Check sheet for the modelled part. Datum: model origin and axes. Units: mm. A direction names the side the tool comes from. Give positions to 0.01 mm unless a question says otherwise; leave off trailing zeros. Order: outer loops, then holes, each group sorted by start corner. A loop starts at its lowest first (then second) coordinate and runs counter-clockwise, first axis right, second up. Notation, with made-up numbers: (-31, 85.25) -> (-18, 85.25) arc R13 cw to (-18, 97.25) -> close; hole circle Ø6 at (12, 36). An arc over 180 degrees is marked (long way). One line per question, with ' | ' between items.
```python
from build123d import *

# Parameters (mm, degrees)
F0_W     = 25
F0_H     = 25
F1_DEPTH = 8.3
F2_R     = 5
F3_DEPTH = 4
F5_DEPTH = 25


with BuildPart() as f1:
    # F0 (on Top) → F1 (new body)
    with BuildSketch(Plane.XY):
        Rectangle(F0_W, F0_H)
    extrude(amount=F1_DEPTH)

    # F2 (on face) → F3 (join)
    with BuildSketch(Plane.XY.offset(8.3)):
        Circle(F2_R)
    extrude(amount=F3_DEPTH)

    # F4 (on face) → F5 (cut)
    with BuildSketch(Plane.XY.offset(8.3)):
        Polygon((12.5, -12.5), (12.5, 0), (0, -12.5), align=None)
    extrude(amount=-F5_DEPTH, mode=Mode.SUBTRACT)


solid = f1.part
```
Q1. Section check B-B (x = -3.5). Enter the section's corners in (y, z).
Result sheet:
outline: (-12.5, 0) -> (12.5, 0) -> (12.5, 8.3) -> (3.57, 8.3) -> (3.57, 12.3) -> (-3.57, 12.3) -> (-3.57, 8.3) -> (-12.5, 8.3) -> close
Q2. Access from +Z, -Z, +X, -X, +Y, -Y to the whole of each face (thin tool, end or side, straight path). Record for faces 1 (the face through (0, 0, 0)), 2 (the face through (-1.08, -4.88, 10.27)).
Result sheet:
face 1: -Z, +X, -X, +Y, -Y | face 2: +Z
Q3. Thickness scan on line 1 (Z direction, x = -0.25, y = -10.25); line 2 (X direction, y = -3.25, z = 9.25); line 3 (Y direction, x = 3, z = 8.25). Record the ranges inside material, lowest first.
Result sheet:
line 1: z = 0 to 8.3 | line 2: x = -3.8 to 3.8 | line 3: y = -9.5 to 12.5
Q4. Section check A-A (z = 4.75). Enter the section's corners in (x, y), and give its area (3 significant figures).
Result sheet:
outline: (-12.5, -12.5) -> (0, -12.5) -> (12.5, 0) -> (12.5, 12.5) -> (-12.5, 12.5) -> close | area: 547 mm2
Q5. Section check C-C (y = 10.75). Enter the section's corners in (x, z), and give its area (4 significant figures).
Result sheet:
outline: (-12.5, 0) -> (12.5, 0) -> (12.5, 8.3) -> (-12.5, 8.3) -> close | area: 207.5 mm2
Q6. Depth check by flat-ended pin: pin 1 Ø1.5 at (y, z) = (-9.5, 6) entering from +X; pin 2 Ø1 at (x, z) = (1.5, 10.5) entering from +Y. Enter the tip coordinate at first touch or a pass-through.
Result sheet:
pin 1: stops at x = 3.75 | pin 2: stops at y = 4.9
